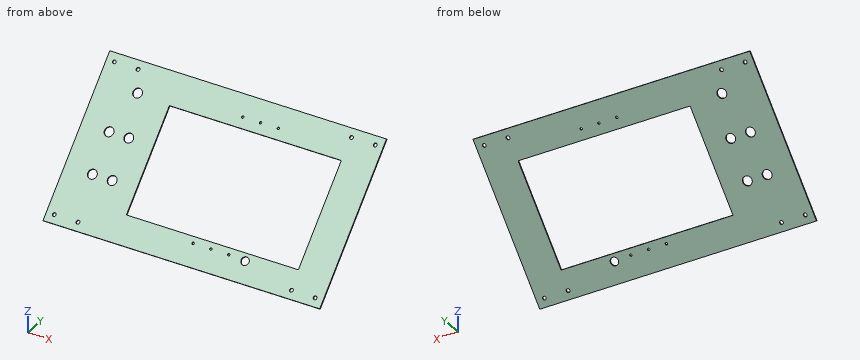
```python
from build123d import *

# Parameters (mm, degrees)
SKETCH034_W          = 700
SKETCH034_H          = 400
SKETCH034_R          = 11.5
SKETCH034_R_2        = 10
SKETCH034_W_2        = 435
SKETCH034_H_2        = 257.5
PAD001_DEPTH         = 3.175
SKETCH044_R          = 2.9
HOLE005_DEPTH        = 25
SKETCH045_R          = 4.5
HOLE006_DEPTH        = 25
BODY_PLACEMENT_ANGLE = 315


with BuildPart() as part:
    # Sketch034 → Pad001 (new body)
    with BuildSketch(Plane.XY):
        with Locations((350, 200)):
            Rectangle(SKETCH034_W, SKETCH034_H)
        with Locations((120, 230)):
            Circle(SKETCH034_R, mode=Mode.SUBTRACT)
        with Locations((100, 330)):
            Circle(SKETCH034_R, mode=Mode.SUBTRACT)
        with Locations((120, 130)):
            Circle(SKETCH034_R, mode=Mode.SUBTRACT)
        with Locations((70, 230)):
            Circle(SKETCH034_R, mode=Mode.SUBTRACT)
        with Locations((490, 50)):
            Circle(SKETCH034_R_2, mode=Mode.SUBTRACT)
        with Locations((70, 130)):
            Circle(SKETCH034_R, mode=Mode.SUBTRACT)
        with Locations((400, 196.25)):
            Rectangle(SKETCH034_W_2, SKETCH034_H_2, mode=Mode.SUBTRACT)
    extrude(amount=-PAD001_DEPTH)

    # Sketch044 → Hole005 (cut)
    with BuildSketch(Plane.XY):
        with Locations((357.5, 350)):
            Circle(SKETCH044_R)
        with Locations((402.5, 350)):
            Circle(SKETCH044_R)
        with Locations((447.5, 350)):
            Circle(SKETCH044_R)
        with Locations((357.5, 52.5)):
            Circle(SKETCH044_R)
        with Locations((402.5, 52.5)):
            Circle(SKETCH044_R)
        with Locations((447.5, 52.5)):
            Circle(SKETCH044_R)
    extrude(amount=-HOLE005_DEPTH, mode=Mode.SUBTRACT)

    # Sketch045 → Hole006 (cut)
    with BuildSketch(Plane.XY):
        with Locations((20, 20)):
            Circle(SKETCH045_R)
        with Locations((680, 20)):
            Circle(SKETCH045_R)
        with Locations((680, 380)):
            Circle(SKETCH045_R)
        with Locations((20, 380)):
            Circle(SKETCH045_R)
        with Locations((80, 20)):
            Circle(SKETCH045_R)
        with Locations((80, 380)):
            Circle(SKETCH045_R)
        with Locations((620, 20)):
            Circle(SKETCH045_R)
        with Locations((620, 380)):
            Circle(SKETCH045_R)
    extrude(amount=-HOLE006_DEPTH, mode=Mode.SUBTRACT)


with BuildPart() as part_1:
    # Body placement: moved
    add(part.part.moved(Location((0, 365, 0))).rotate(Axis((0, 365, 0), (-1, 0, 0)), BODY_PLACEMENT_ANGLE))


solid = part_1.part
```
Work out the finished part from the listing and answer in its coordinate system (mm). Give positions to 0.01 mm unless a question says otherwise; leave off trailing zeros. Order: outer loops, then holes, each group sorted by start corner. A loop starts at its lowest first (then second) coordinate and runs counter-clockwise, first axis right, second up. Notation, with made-up numbers: (-10.75, -20) -> (1.25, -20) arc R18 cw to (1.25, 12) -> close; hole circle Ø8 at (32.25, 41.5). An arc over 180 degrees is marked (long way). Answer as CSV lines item,"result". Start each with the question number.
(1) Section A-A, the plane x = 240.5 is taken. Write down the section's boundary in (y, z).
(2) Each of these flat-tipped pins is pushed along its axis until it touches: pin 1 Ø10 at (x, z) = (110, 227.5) entering from -Y; pin 2 Ø3 at (x, y) = (128.5, 518.5) entering from -Z. Where does it stop, or does it pass through?
(3) Section B-B, the plane z = 192.5 is taken. Write down the section's boundary in (x, y).
(4) Consider line 1 along Z through (x, y) = (211.5, 634); line 2 along Z through (x, y) = (370.5, 412); line 3 along Y through (x, z) = (127, 230.5). Determine where each line is inside the solid, lowest interval first.
Entries:
1,outline,"(365, 0) -> (367.25, -2.25) -> (414.97, 45.48) -> (412.73, 47.73) -> close; (594.81, 229.81) -> (597.05, 227.56) -> (650.09, 280.6) -> (647.84, 282.84) -> close"
2,pin 1,"y = 587.5"
2,pin 2,"z = 147.51"
3,outline,"(0, 557.5) -> (182.5, 557.5) -> (182.5, 561.99) -> (0, 561.99) -> close; (617.5, 557.5) -> (700, 557.5) -> (700, 561.99) -> (617.5, 561.99) -> close"
4,line 1,"264.51 to 269"
4,line 2,"42.51 to 47"
4,line 3,"595.5 to 599.99"
